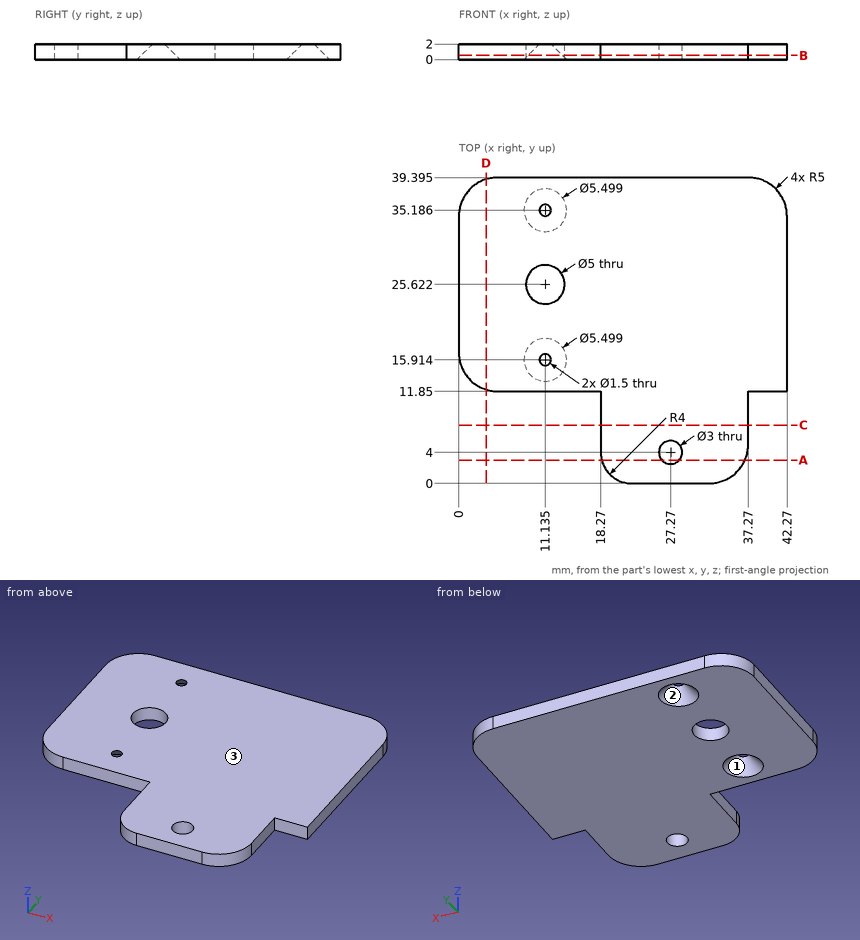
Can you work these out from the drawing? Everything is in mm from the part's minimum corner. Round coordinates to 2 decimals unless told otherwise and drop trailing zeros. Loops run counter-clockwise (first coordinate to the right, second up) from the corner with the lowest first, then second, coordinate; pieces in that order, holes last. Notation, with made-up numbers: (48, -34.75) - (68, -34.75) arc R10 ccw to (68, -22.75) - close; hole circle Ø6 at (60.25, 82.5). An arc over 180 degrees is marked (long way). Answer in a Markdown table with one row per item. Add a question column.
Q1. I want a section at A-A on y = 3. List the corners of the cut face in (x, z) for me.
Q2. I need wall thicknesses on L1, parallel to X at y = 25.5, z = 0.55; L2, parallel to X at y = 14.5, z = 0.2 (1 decimal); L3, parallel to X at y = 11.5, z = 1.3. Which ranges of each line are inside material? Lowest first, please.
Q3. I want a section at C-C on y = 7.5. List the corners of the cut face in (x, z) for me.
Q4. I want a section at B-B on z = 0.55. Count the separate pieces of the cut face and the enclosed holes in it, and give its area (3 significant figures).
Q5. We'd pull the mould along X, two halves only. Please class the marked faces 1, 2 and 3: pulls with the +X half, pulls with the -X half, needs draft (parallel to the pull), parting line crosses it, or undercut.
Q6. For pin 1 Ø0.6 at (y, z) = (7, 1) entering from +X, with a flat end and sliding along its axis, tell me the tip position at first contact or that it passes through.
Q7. I want a section at D-D on x = 3.5. List the corners of the cut face in (y, z) for me (1 decimal).
A:
| question | item | result |
|---|---|---|
| 1 | outline | (18.4, 0) - (26.15, 0) - (26.15, 2) - (18.4, 2) - close; (28.39, 0) - (36.85, 0) - (36.85, 2) - (28.39, 2) - close |
| 2 | L1 | 0 to 8.64, 13.63 to 42.27 |
| 2 | L2 | 0.6 to 9, 13.3 to 42.3 |
| 2 | L3 | 18.27 to 37.27 |
| 3 | outline | (18.27, 0) - (37.27, 0) - (37.27, 2) - (18.27, 2) - close |
| 4 | separate pieces | 1 |
| 4 | enclosed holes | 4 |
| 4 | area | 1,310 mm^2 |
| 5 | face 1 | undercut |
| 5 | face 2 | undercut |
| 5 | face 3 | needs draft |
| 6 | pin 1 | x = 37.27 |
| 7 | outline | (12.1, 0) - (39.2, 0) - (39.2, 2) - (12.1, 2) - close |
